from build123d import *


with BuildPart() as part:
    # BodySke → Body (revolve)
    with BuildSketch(Plane.XY, mode=Mode.PRIVATE) as body_sk:
        with BuildLine():
            Line((4.6, 8), (58, 8))
            Line((58, 8), (60, 7.464101615))
            Line((60, 7.464101615), (60, 5.25))
            Line((60, 5.25), (58.5, 5.25))
            Line((58.5, 5.25), (57.431902002, 3.4))
            Line((57.431902002, 3.4), (35, 3.4))
            Line((35, 3.4), (33.591673888, 0))
            Line((33.591673888, 0), (0, 0))
            ThreePointArc((0, 0), (0.437676073, 3.716728939), (1.726759251, 7.230117462))
            Line((1.726759251, 7.230117462), (4.6, 8))
        make_face()
    revolve(body_sk.sketch.rotate(Axis((0, 0, 0), (1, 0, 0)), 90), axis=Axis((0, 0, 0), (1, 0, 0)))


solid = part.part
Part model, mm, in its own coordinate system. A direction names the side the tool comes from. Round coordinates to 2 decimals unless told otherwise and drop trailing zeros. Loops run counter-clockwise (first coordinate to the right, second up) from the corner with the lowest first, then second, coordinate; pieces in that order, holes last. Notation, with made-up numbers: (18.25, -2) - (53.25, -2) arc R22 cw to (53.25, 6) - close; hole circle Ø1 at (-32, -32.75). An arc over 180 degrees is marked (long way). Answer as a JSON object with one key per item and string values.
Item 1: Pin check, flat tips, straight feed: pin 1 (1.5 mm diameter, centred on x = 36, y = -4, fed in from -Z); pin 2 (3 mm diameter, centred on x = 45.5, y = -3.5, fed in from +Z); pin 3 (1 mm diameter, centred on x = 8.5, z = -5.5, fed in from +Y) (3 decimals). Stop position of each tip, or through.
Output:
{"pin 1": "z = -7.31", "pin 2": "z = 7.75", "pin 3": "y = 6.245"}
Item 2: Band-saw the part on B-B on x = 43. List the corners of the cut face in (y, z).
Output:
{"outline": "circle Ø16 at (0, 0); hole circle Ø6.8 at (0, 0)"}
Item 3: Tool access for faces 4 (the face through (46.06, 3.32, -0.74)), 5 (the face through (31.67, 7.81, -1.73)): list every direction of +Z, -Z, +X, -X, +Y, -Y with a clear straight run to the whole face (end or side of a thin tool).
Output:
{"face 4": "+X", "face 5": "+X, -X"}
Item 4: Band-saw the part on A-A on x = 7. List the corners of the cut face in (y, z), plus the area to 3 significant figures.
Output:
{"outline": "circle Ø16 at (0, 0)", "area": "201 mm2"}
Item 5: Wall check: L1, parallel to Y at x = 46, z = 0; L2, parallel to Y at x = 58.95, z = 0; L3, parallel to X at y = 3.5, z = -0.5. Give the ranges that are in metal, low to high.
Output:
{"L1": "-8 to -3.4, 3.4 to 8", "L2": "-7.75 to -5.25, 5.25 to 7.75", "L3": "0.4 to 57.51"}
Item 6: Pull direction Y, two halves, no side cores. Call faces 1 (the face through (60, -5.1, -1.8)), 2 (the face through (1.91, -2.19, 6.94)), 3 (the face through (59.2, -1.6, 5)): pulls with the +Y half, pulls with the -Y half, needs draft (parallel to the pull), parting line crosses it, or undercut.
Output:
{"face 1": "needs draft", "face 2": "parting line crosses it", "face 3": "undercut"}
